Source: CAD feature listing. Evaluate the final solid. Frame: model axes, mm. Give positions to 0.01 mm unless a question says otherwise; leave off trailing zeros. Order: outer loops, then holes, each group sorted by start corner. A loop starts at its lowest first (then second) coordinate and runs counter-clockwise, first axis right, second up. Notation, with made-up numbers: (-33.5, 40) - (-18.5, 40) arc R18 ccw to (-18.5, 45) - close; hole circle Ø8 at (-12.75, -35). An arc over 180 degrees is marked (long way). Write each question's results on one line, items separated by ' | '. Start each with the question number.
Item 1: Line query: line 1 along Z through (x, y) = (14, 0.5); line 2 along Y through (x, z) = (6, 34); line 3 along X through (y, z) = (16, 17). Output: solid intervals per line, ascending.
Item 2: Mould query, pull axis Z, two halves, no side actions, for faces 1 (the cylindrical face through (14.881, -5.073, 12.525)), 2 (the flat face through (0, 6, 0)), 3 (the cylindrical face through (32.816, -19.854, 25.044)). Classes: released by +Z, released by -Z, zero draft, split by the parting line, or undercut.
Item 3: Contact query for flat-ended pins moving along their axis: pin 1 Ø6 at (y, z) = (16, 13.5) entering from -X; pin 2 Ø3 at (y, z) = (17.5, 20.5) entering from -X; pin 3 Ø6 at (x, z) = (4, 26) entering from -Y. Output: stop coordinate, or through.
Item 4: Section B-B on y = 17.5. Output: boundary loops of the cut face in (x, z).
Item 5: Section C-C on x = -19.5. Output: boundary loops of the cut face in (y, z), and give its area (3 significant figures).
```python
from build123d import *

# Parameters (mm, degrees)
F1_DEPTH = 50.8
F4_R     = 5.08
F5_DEPTH = 63.5


with BuildPart() as f1:
    # F0 (on Top) → F1 (new body)
    with BuildSketch(Plane.XY):
        with BuildLine():
            ThreePointArc((12.7995573241, -1.6389246221), (17.4709677584, 4.1647671705), (24.5934442484, 6.35))
            ThreePointArc((24.5934442484, 6.35), (-6.35, 24.5934442484), (-24.5934442484, -6.35))
            ThreePointArc((-24.5934442484, -6.35), (-6.35, -0.3984375242), (12.7995573241, -1.6389246221))
        make_face()
        with BuildLine():
            ThreePointArc((12.7995573241, -1.6389246221), (-6.35, -0.3984375242), (-24.5934442484, -6.35))
            ThreePointArc((-24.5934442484, -6.35), (-6.35, -24.5934442484), (18.4450831863, -17.4625))
            ThreePointArc((18.4450831863, -17.4625), (12.6319455908, -10.6176164148), (12.7995573241, -1.6389246221))
        make_face()
        with BuildLine():
            ThreePointArc((18.4450831863, -17.4625), (22.225, -12.2967221242), (24.5934442484, -6.35))
            ThreePointArc((24.5934442484, -6.35), (18.8443015114, -3.6244523026), (12.7995573241, -1.6389246221))
            ThreePointArc((12.7995573241, -1.6389246221), (12.6319455908, -10.6176164148), (18.4450831863, -17.4625))
        make_face()
        with BuildLine():
            ThreePointArc((24.5934442484, -6.35), (25.1975542852, -3.2005090291), (25.4, 0))
            ThreePointArc((25.4, 0), (25.1975542852, 3.2005090291), (24.5934442484, 6.35))
            ThreePointArc((24.5934442484, 6.35), (17.4709677584, 4.1647671705), (12.7995573241, -1.6389246221))
            ThreePointArc((12.7995573241, -1.6389246221), (18.8443015114, -3.6244523026), (24.5934442484, -6.35))
        make_face()
        with BuildLine():
            ThreePointArc((24.5934442484, 6.35), (25.1975542852, 3.2005090291), (25.4, 0))
            ThreePointArc((25.4, 0), (25.1975542852, -3.2005090291), (24.5934442484, -6.35))
            ThreePointArc((24.5934442484, -6.35), (27.3340357189, -7.9807229005), (29.9669059095, -9.7801931963))
            ThreePointArc((29.9669059095, -9.7801931963), (33.2813397987, -7.6860670857), (37.1938348674, -7.9375))
            ThreePointArc((37.1938348674, -7.9375), (37.2685174407, -7.1453109893), (37.2934442484, -6.35))
            ThreePointArc((37.2934442484, -6.35), (33.5737003695, 2.6302561211), (24.5934442484, 6.35))
        make_face()
        with BuildLine():
            ThreePointArc((29.9669059095, -9.7801931963), (27.3340357189, -7.9807229005), (24.5934442484, -6.35))
            ThreePointArc((24.5934442484, -6.35), (22.225, -12.2967221242), (18.4450831863, -17.4625))
            ThreePointArc((18.4450831863, -17.4625), (24.1451446263, -19.0420852286), (29.9424477824, -17.8686006613))
            ThreePointArc((29.9424477824, -17.8686006613), (28.5002699382, -13.8199990211), (29.9669059095, -9.7801931963))
        make_face()
        with BuildLine():
            ThreePointArc((34.8502409072, -13.8392003779), (32.4720574524, -11.7333200181), (29.9669059095, -9.7801931963))
            ThreePointArc((29.9669059095, -9.7801931963), (28.5002699382, -13.8199990211), (29.9424477824, -17.8686006613))
            ThreePointArc((29.9424477824, -17.8686006613), (32.6522448152, -16.1655862497), (34.8502409072, -13.8392003779))
        make_face()
        with BuildLine():
            ThreePointArc((37.1938348674, -7.9375), (33.2813397987, -7.6860670857), (29.9669059095, -9.7801931963))
            ThreePointArc((29.9669059095, -9.7801931963), (32.4720574524, -11.7333200181), (34.8502409072, -13.8392003779))
            ThreePointArc((34.8502409072, -13.8392003779), (36.3968450041, -11.0371879203), (37.1938348674, -7.9375))
        make_face()
        with BuildLine():
            ThreePointArc((41.2002409072, -13.8392003779), (40.1040167707, -10.272641928), (37.1938348674, -7.9375))
            ThreePointArc((37.1938348674, -7.9375), (36.3968450041, -11.0371879203), (34.8502409072, -13.8392003779))
            ThreePointArc((34.8502409072, -13.8392003779), (35.9893415804, -14.9474227898), (37.0932189983, -16.0907346038))
            ThreePointArc((37.0932189983, -16.0907346038), (38.9431027022, -15.3102596751), (40.8913363289, -15.7956425842))
            ThreePointArc((40.8913363289, -15.7956425842), (41.1225393666, -14.829539732), (41.2002409072, -13.8392003779))
        make_face()
        with BuildLine():
            ThreePointArc((34.8502409072, -13.8392003779), (32.6522448152, -16.1655862497), (29.9424477824, -17.8686006613))
            ThreePointArc((29.9424477824, -17.8686006613), (32.8633256958, -19.8703418903), (36.4020454568, -19.9966676039))
            ThreePointArc((36.4020454568, -19.9966676039), (36.0626125115, -17.922483586), (37.0932189983, -16.0907346038))
            ThreePointArc((37.0932189983, -16.0907346038), (35.9893415804, -14.9474227898), (34.8502409072, -13.8392003779))
        make_face()
        with BuildLine():
            ThreePointArc((37.0932189983, -16.0907346038), (36.0626125115, -17.922483586), (36.4020454568, -19.9966676039))
            ThreePointArc((36.4020454568, -19.9966676039), (37.892136008, -19.4131912458), (39.1890408908, -18.4757200535))
            ThreePointArc((39.1890408908, -18.4757200535), (38.1597671946, -17.2668497207), (37.0932189983, -16.0907346038))
        make_face()
        with BuildLine():
            ThreePointArc((40.8913363289, -15.7956425842), (38.9431027022, -15.3102596751), (37.0932189983, -16.0907346038))
            ThreePointArc((37.0932189983, -16.0907346038), (38.1597671946, -17.2668497207), (39.1890408908, -18.4757200535))
            ThreePointArc((39.1890408908, -18.4757200535), (40.2103958459, -17.243791254), (40.8913363289, -15.7956425842))
        make_face()
        with BuildLine():
            ThreePointArc((42.3640408908, -18.4757200535), (41.971612814, -16.9466947129), (40.8913363289, -15.7956425842))
            ThreePointArc((40.8913363289, -15.7956425842), (40.2103958459, -17.243791254), (39.1890408908, -18.4757200535))
            ThreePointArc((39.1890408908, -18.4757200535), (40.1800346913, -19.7161647764), (41.1317805923, -20.9869722217))
            ThreePointArc((41.1317805923, -20.9869722217), (42.0393762704, -19.8743669796), (42.3640408908, -18.4757200535))
        make_face()
        with BuildLine():
            ThreePointArc((39.1890408908, -18.4757200535), (37.892136008, -19.4131912458), (36.4020454568, -19.9966676039))
            ThreePointArc((36.4020454568, -19.9966676039), (38.5383737374, -21.583332844), (41.1317805923, -20.9869722217))
            ThreePointArc((41.1317805923, -20.9869722217), (40.1800346913, -19.7161647764), (39.1890408908, -18.4757200535))
        make_face()
    extrude(amount=F1_DEPTH)

    # F4 (on 3pt) → F5 (cut, symmetric)
    with BuildSketch(Plane(origin=(36.3446660233, -9.3841524154, 17.0086899215), x_dir=(0.2062459752, 0.9737281746, 0.0965196334), z_dir=(0.8819306257, -0.2277135084, 0.4127286391))):
        Circle(F4_R)
    extrude(amount=F5_DEPTH, both=True, mode=Mode.SUBTRACT)


solid = f1.part
```
Evaluation:
1) line 1: z = 0 to 2.63, 9.55 to 50.8 | line 2: y = -24.68 to 24.68 | line 3: x = -19.73 to 19.73
2) face 1: undercut | face 2: released by -Z | face 3: zero draft
3) pin 1: stops at x = -21.82 | pin 2: stops at x = -19.73 | pin 3: stops at y = -25.38
4) outline: (-18.41, 0) - (18.41, 0) - (18.41, 50.8) - (-18.41, 50.8) - close
5) outline: (-16.28, 0) - (16.28, 0) - (16.28, 50.8) - (-16.28, 50.8) - close | area: 1,650 mm^2
